Could you check a few things on this model? Use its own coordinates, in mm. A direction names the side the tool comes from. Coordinates: 2 decimals unless noted, no trailing zeros. Loops run counter-clockwise (first coordinate to the right, second up) from the corner with the lowest first, then second, coordinate; pieces in that order, holes last. Notation, with made-up numbers: M 63,43 L 115,43 A35 cw 115,79 Z; hole C 9.5,6 d7. An arc over 180 degrees is marked long. Write each question's results on one line, items separated by ' | '.
```python
from build123d import *

# Parameters (mm, degrees)
SKETCH002_AS_DRAWN_R                 = 1.65
EXTRUDE003_DEPTH                     = 6
EXTRUDE003_ONTO_SKETCH002_ROLL_ANGLE = 90
SKETCH003_R                          = 3.1
PAD_DEPTH                            = 5
PAD001_DEPTH                         = 5
EXTRUDE_DEPTH                        = 1
EXTRUDE002_DEPTH                     = 7


with BuildPart() as body:
    # Sketch002 as drawn → Extrude003 (new, symmetric)
    with BuildSketch(Plane.XY):
        with Locations((-5.676932, 4.1)):
            Circle(SKETCH002_AS_DRAWN_R)
    extrude(amount=EXTRUDE003_DEPTH, both=True)


with BuildPart() as body_1:
    # Extrude003 onto Sketch002 roll: moved
    add(body.part.rotate(Axis((0, 0, 0), (1, 0, 0)), EXTRUDE003_ONTO_SKETCH002_ROLL_ANGLE))


with BuildPart() as body_2:
    # Extrude003 onto Sketch002 placement: moved
    add(body_1.part)

    # Sketch003 (on Face3 of BaseFeature) → Pad (new body)
    with BuildSketch(Plane.XZ.offset(6)):
        with Locations((-5.676932, 4.1)):
            Circle(SKETCH003_R)
    extrude(amount=PAD_DEPTH)

    # Sketch004 (on Face1 of Pad) → Pad001 (join)
    with BuildSketch(Plane(origin=(0, 6, 0), x_dir=(-1, 0, 0), z_dir=(0, 1, 0))):
        Polygon((5.676932, 0.797556), (8.536932, 2.448778), (8.536932, 5.751222), (5.676932, 7.402444), (2.816932, 5.751222), (2.816932, 2.448778), align=None)
    extrude(amount=PAD001_DEPTH)


with BuildPart() as extrude001:
    # Sketch001 → Extrude (new body)
    with BuildSketch(Plane.XY):
        Polygon((0, 0), (-15, 0), (-15, 15.001059), (5.758367, 15.001059), align=None)
    extrude(amount=EXTRUDE_DEPTH)


with BuildPart() as cut001:
    # Sketch → Extrude002 (new body)
    with BuildSketch(Plane.XY):
        with BuildLine():
            ThreePointArc((-2.478407, -0.6), (2.55, 0), (-2.478407, 0.6))
            Line((-8.978407, 0.6), (-2.478407, 0.6))
            Line((-8.978407, 0.6), (-8.978407, 7.002256))
            ThreePointArc((-8.478407, 7.6), (-8.733522, 7.305407), (-8.978407, 7.002256))
            Line((-8.478407, 7.6), (-2.497999, 7.6))
            ThreePointArc((-2.497999, -7.6), (8, 0), (-2.497999, 7.6))
            Line((-8.478407, -7.6), (-2.497999, -7.6))
            ThreePointArc((-8.978407, -7.002256), (-8.733522, -7.305407), (-8.478407, -7.6))
            Line((-8.978407, -0.6), (-8.978407, -7.002256))
            Line((-8.978407, -0.6), (-2.478407, -0.6))
        make_face()
    extrude(amount=EXTRUDE002_DEPTH)

    # Cut: cut Extrude001
    add(extrude001.part, mode=Mode.SUBTRACT)

    # Cut001: cut Body
    add(body_2.part, mode=Mode.SUBTRACT)


solid = cut001.part
```
(1) Imagine slicing it at C-C, the plane y = 3. List the corners of the cut face in (x, z) for me.
Reported:
outline: M -8.98,1 L 1.15,1 L 1.15,0 L 7.42,0 L 7.42,7 L -8.98,7 Z; hole C -5.68,4.1 d3.3
(2) Please list where these lines run through material, in increasing order: probe 1 along Y at (x, z) = (0, 2.75); probe 2 along Y at (x, z) = (-3, 3); probe 3 along Z at (x, y) = (-0.5, 3). Write a range as from..to.
Reported:
probe 1: y = -8..-2.55, 2.55..8 | probe 2: y = -6..-0.6, 0.6..6 | probe 3: z = 1..7
(3) Imagine slicing it at A-A, the plane x = 0. List the corners of the cut face in (y, z) for me, and give its area (4 significant figures).
Reported:
outline: M -8,0 L -2.55,0 L -2.55,7 L -8,7 Z; M 2.55,1 L 8,1 L 8,7 L 2.55,7 Z | area: 70.85 mm2
(4) Imagine slicing it at D-D, the plane z = 3.5. List the corners of the cut face in (x, y) for me, and give its area (3 significant figures).
Reported:
outline: M -8.98,-7 A11.39 ccw -8.72,-7.32 L -8.72,-6 L -7.21,-6 L -7.21,-0.6 L -8.98,-0.6 Z; M -8.98,0.6 L -7.21,0.6 L -7.21,6 L -8.54,6 L -8.54,7.53 A11.39 ccw -8.98,7 Z; M -4.14,-6 L -2.64,-6 L -2.64,-7.6 L -2.5,-7.6 A8 ccw long -2.5,7.6 L -2.82,7.6 L -2.82,6 L -4.14,6 L -4.14,0.6 L -2.48,0.6 A2.55 cw long -2.48,-0.6 L -4.14,-0.6 Z | area: 158 mm2
(5) Imagine slicing it at B-B, the plane y = -1.25. List the corners of the cut face in (x, z) for me, and give its area (3 significant figures).
Reported:
outline: M -8.98,0 L -2.22,0 L -2.22,7 L -8.98,7 Z; M 2.22,0 L 7.9,0 L 7.9,7 L 2.22,7 Z; hole C -5.68,4.1 d3.3 | area: 78.5 mm2
(6) Will these pins go through, and if not, where does the flat tip stop? P1, Ø8, axis at x = -5.5, y = 5.5, coming from the -Z side; P2, Ø2.5, axis at x = -5.68, z = 4.1, coming from the +Y side (1 decimal); P3, Ø1.2, axis at y = 6.5, z = 3.5, coming from the +X side; P4, Ø1.8, axis at x = -6, z = 2, coming from the -Y side.
Reported:
P1: stops at z = 1 | P2: passes through | P3: stops at x = 5.4 | P4: stops at y = -6
(7) If we mould it in two halves opening along Y, with no side actions, what happens to faces 4 (the cylindrical face through (2.55, -0.1, 3.45)), 5 (the flat face through (-3.91, 6.79, 6.38)), 6 (the flat face through (-4, 6, 5)), 7 (the flat face through (-6, -0.6, 2))? For each: released by +Y, released by -Y, zero draft, split by the parting line, or undercut.
Reported:
face 4: undercut | face 5: zero draft | face 6: released by +Y | face 7: undercut
(8) Which directions (+Z, -Z, +X, -X, +Y, -Y) give clear straight access to the entire face, cutting with the end or side of a thin tool? Please do faces 1 (the flat face through (-2.817, 7, 4)), 2 (the flat face through (-7.2, 0.6, 2.6)), 3 (the flat face through (1.904, 4.96, 0.493)).
Reported:
face 1: +Y | face 2: +Z, -Z, -X | face 3: -Z, -X, +Y
